Read the model definition and answer for the solid it produces. Units are mm, in the model's axes. Face numbers are marked on the shaded views. A direction names the side the tool comes from. Give positions to 0.01 mm unless a question says otherwise; leave off trailing zeros. Write each loop counter-clockwise with the first axis right and the second up, starting at its lowest first coordinate (ties: lowest second). Pieces come first, ordered by that corner, then holes. Notation, with made-up numbers: M -15,11 L 36,11 A19 ccw 36,40 Z; hole C 50,28.25 d3. An arc over 180 degrees is marked long. Use a Markdown table: item, result. Add a question column.
Item 1: A cutting plane is placed at D-D on y = -9.5. Determine the outline of the cut face in (x, z).
Item 2: A cutting plane is placed at C-C on y = 8.5. Determine the outline of the cut face in (x, z).
Item 3: Consider probe 1 along X at (y, z) = (-6, 27); probe 2 along X at (y, z) = (48.26, -149.75); probe 3 along Y at (x, z) = (76, 15). Determine where each line is inside the solid, lowest interval first. Write a range as [from, to].
Item 4: A cutting plane is placed at B-B on y = 48.26. Determine the outline of the cut face in (x, z).
Item 5: The mould has two halves that part along X. Classify the marked faces 4, 5 and 6: pulls with the +X half, pulls with the -X half, needs draft (parallel to the pull), parting line crosses it, or undercut.
Item 6: A cutting plane is placed at A-A on x = 0. Determine the outline of the cut face in (y, z), then the cut area to 3 significant figures.
Item 7: Given P1, Ø22.5, axis at x = 40.5, y = 53.5, coming from the +Z side; P2, Ø2, axis at x = 0.5, y = 5, coming from the -Z side; P3, Ø1.9, axis at x = 2, y = 10.5, coming from the -Z side; P4, Ø11.5, axis at x = 0, y = -6.35, coming from the +Z side, each flat-ended and moving along its own axis, determine where each tip first touches the part or whether it passes through.
Item 8: For the marked faces 1, 2 and 3, determine the directions among +Z, -Z, +X, -X, +Y, -Y from which every point of the face is accessible in a straight line to the end or side of a thin tool.
from build123d import *

# Parameters (mm, degrees)
SKETCH1_W               = 177.8
SKETCH1_H               = 101.6
BOSS_EXTRUDE1_DEPTH     = 12.7
SKETCH2_W               = 25.4
SKETCH2_H               = 19.05
BOSS_EXTRUDE2_DEPTH     = 101.6
SKETCH3_R               = 6.35
CUT_EXTRUDE1_DEPTH      = 101.6
SKETCH4_W               = 25.4
SKETCH4_H               = 19.05
BOSS_EXTRUDE3_DEPTH     = 101.6
SKETCH5_R               = 6.35
CUT_EXTRUDE2_DEPTH      = 101.6
SKETCH6_W               = 76.2
SKETCH6_H               = 31.75
CUT_EXTRUDE3_DEPTH      = 101.6
FILLET1_R               = 6.35
SKETCH8_W               = 101.6
SKETCH8_H               = 12.7
BOSS_EXTRUDE5_DEPTH     = 85.09
SKETCH9_W               = 40.7
SKETCH9_H               = 68.61
SKETCH9_R               = 6
BOSS_EXTRUDE6_DEPTH     = 16.35
SKETCH10_R              = 14
CUT_EXTRUDE4_DEPTH      = 10
FILLET2_R               = 6.35
SKETCH11_W              = 105.926535366
SKETCH11_H              = 109.219193109
CUT_EXTRUDE5_DEPTH      = 6.35
FILLET3_R               = 3.175
SKETCH12_W              = 101.6
SKETCH12_H              = 25.4
CUT_EXTRUDE6_DEPTH      = 3.175
CUT_EXTRUDE6_DEPTH_BACK = 39.25


with BuildPart() as part:
    # Sketch1 → Boss-Extrude1 (new body)
    with BuildSketch(Plane(origin=(0, 0, 0), x_dir=(1, 0, 0), z_dir=(0, 1, 0))):
        Rectangle(SKETCH1_W, SKETCH1_H)
    extrude(amount=BOSS_EXTRUDE1_DEPTH)

    # Sketch2 → Boss-Extrude2 (add)
    with BuildSketch(Plane.XY.offset(50.8)):
        with Locations((0, -9.525)):
            Rectangle(SKETCH2_W, SKETCH2_H)
    extrude(amount=-BOSS_EXTRUDE2_DEPTH)

    # Sketch3 → Cut-Extrude1 (cut)
    with BuildSketch(Plane.XY.offset(50.8)):
        with Locations((0, -6.35)):
            Circle(SKETCH3_R)
    extrude(amount=-CUT_EXTRUDE1_DEPTH, mode=Mode.SUBTRACT)

    # Sketch4 → Boss-Extrude3 (add)
    with BuildSketch(Plane.XY.offset(50.8)):
        with Locations((-76.2, -9.525)):
            Rectangle(SKETCH4_W, SKETCH4_H)
    boss_extrude3 = extrude(amount=-BOSS_EXTRUDE3_DEPTH)

    # Mirror1: Boss-Extrude3 across plane
    add(boss_extrude3.mirror(Plane(origin=(0, 0, 0), x_dir=(0, 0, 1), z_dir=(1, 0, 0))))

    # Sketch5 → Cut-Extrude2 (cut)
    with BuildSketch(Plane.XY.offset(50.8)):
        with Locations((-76.2, -6.35)):
            Circle(SKETCH5_R)
        with Locations((76.2, -6.35)):
            Circle(SKETCH5_R)
    extrude(amount=-CUT_EXTRUDE2_DEPTH, mode=Mode.SUBTRACT)

    # Sketch6 → Cut-Extrude3 (cut)
    with BuildSketch(Plane(origin=(0, 0, -50.8), x_dir=(-1, 0, 0), z_dir=(0, 0, -1))):
        with Locations((50.8, -3.175)):
            Rectangle(SKETCH6_W, SKETCH6_H)
    extrude(amount=-CUT_EXTRUDE3_DEPTH, mode=Mode.SUBTRACT)

    # Fillet1
    fillet1_edges = [part.edges().sort_by_distance(p)[0] for p in [
        (12.7, 0, 0),
        (63.5, 0, 0),
    ]]
    fillet(fillet1_edges, radius=FILLET1_R)

    # Sketch8 → Boss-Extrude5 (add)
    with BuildSketch(Plane(origin=(0, 0, -50.8), x_dir=(-1, 0, 0), z_dir=(0, 0, -1))):
        with Locations((-38.1, 6.35)):
            Rectangle(SKETCH8_W, SKETCH8_H)
    extrude(amount=BOSS_EXTRUDE5_DEPTH)

    # Sketch9 → Boss-Extrude6 (add)
    with BuildSketch(Plane(origin=(0, 0, -135.89), x_dir=(-1, 0, 0), z_dir=(0, 0, -1))):
        with Locations((-38.1, 34.305)):
            Rectangle(SKETCH9_W, SKETCH9_H)
        with Locations((-38.1, 48.26)):
            Circle(SKETCH9_R, mode=Mode.SUBTRACT)
    extrude(amount=BOSS_EXTRUDE6_DEPTH)

    # Sketch10 → Cut-Extrude4 (cut)
    with BuildSketch(Plane.XY.offset(-135.89)):
        with Locations((38.1, 48.26)):
            Circle(SKETCH10_R)
    extrude(amount=-CUT_EXTRUDE4_DEPTH, mode=Mode.SUBTRACT)

    # Fillet2
    fillet2_edges = [part.edges().sort_by_distance(p)[0] for p in [
        (58.45, 6.35, -135.89),
        (17.75, 6.35, -135.89),
    ]]
    fillet(fillet2_edges, radius=FILLET2_R)

    # Sketch11 → Cut-Extrude5 (cut)
    with BuildSketch(Plane.XZ):
        with Locations((35.936732317, -105.409596555)):
            Rectangle(SKETCH11_W, SKETCH11_H)
    extrude(amount=-CUT_EXTRUDE5_DEPTH, mode=Mode.SUBTRACT)

    # Fillet3
    fillet3_edges = [part.edges().sort_by_distance(p)[0] for p in [
        (38.1, 6.35, -50.8),
    ]]
    fillet(fillet3_edges, radius=FILLET3_R)

    # Sketch12 → Cut-Extrude6 (cut, two sides)
    with BuildSketch(Plane(origin=(0, 0, -50.8), x_dir=(-1, 0, 0), z_dir=(0, 0, -1))) as cut_extrude6_sk:
        with Locations((-38.1, -6.35)):
            Rectangle(SKETCH12_W, SKETCH12_H)
    extrude(amount=CUT_EXTRUDE6_DEPTH, mode=Mode.SUBTRACT)
    extrude(cut_extrude6_sk.sketch, amount=-CUT_EXTRUDE6_DEPTH_BACK, mode=Mode.SUBTRACT)


solid = part.part
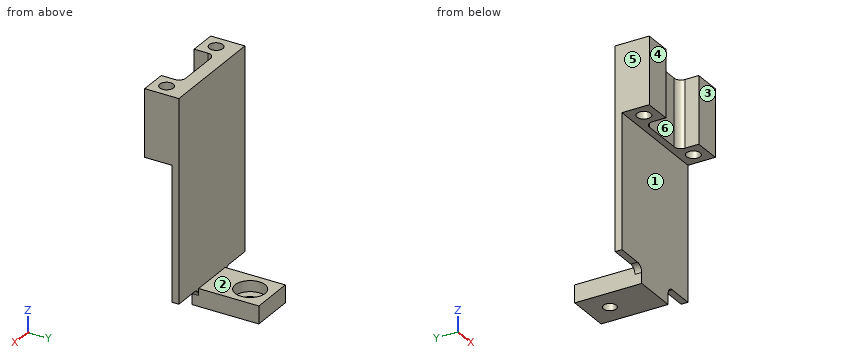
Filled in:
| question | item | result |
|---|---|---|
| 1 | outline | M -12.7,-11.55 L -5.51,-11.55 L -5.51,50.8 L -12.7,50.8 Z; M 5.51,-11.55 L 12.7,-11.55 L 12.7,50.8 L 5.51,50.8 Z; M 63.5,-11.55 L 70.69,-11.55 L 70.69,50.8 L 63.5,50.8 Z; M 81.71,-11.55 L 88.9,-11.55 L 88.9,50.8 L 81.71,50.8 Z |
| 2 | outline | M -12.7,-135.89 L 11.4,-135.89 A6.35 cw 17.75,-142.24 L 17.75,-152.24 L 58.45,-152.24 L 58.45,-142.24 A6.35 cw 64.8,-135.89 L 88.9,-135.89 L 88.9,50.8 L -12.7,50.8 Z |
| 3 | probe 1 | [-12.7, -6.34], [6.34, 12.71], [63.49, 69.86], [82.54, 88.9] |
| 3 | probe 2 | [17.75, 32.1], [44.1, 58.45] |
| 3 | probe 3 | [-19.05, -12.7], [0, 12.7] |
| 4 | outline | M 17.75,-152.24 L 32.1,-152.24 L 32.1,-145.89 L 24.1,-145.89 L 24.1,-135.89 L 17.75,-135.89 Z; M 44.1,-152.24 L 58.45,-152.24 L 58.45,-135.89 L 52.1,-135.89 L 52.1,-145.89 L 44.1,-145.89 Z |
| 5 | face 4 | needs draft |
| 5 | face 5 | pulls with the -X half |
| 5 | face 6 | undercut |
| 6 | outline | M -19.05,-11.55 L -12.7,-11.55 L -12.7,50.8 L -19.05,50.8 Z; M 0,-11.55 L 6.35,-11.55 L 6.35,-135.89 L 12.7,-135.89 L 12.7,50.8 L 0,50.8 Z |
| 6 | area | 1,980 mm² |
| 7 | P1 | z = -135.89 |
| 7 | P2 | z = -11.55 |
| 7 | P3 | z = -135.89 |
| 7 | P4 | through |
| 8 | face 1 | -Z, +X, -X, -Y |
| 8 | face 2 | +Z, +X, -X, +Y |
| 8 | face 3 | +Z, -Z, +X, -X, -Y |
